Could you check a few things on this model? Use its own coordinates, in mm. Face numbers are marked on the shaded views. Round coordinates to 2 decimals unless told otherwise and drop trailing zeros. Loops run counter-clockwise (first coordinate to the right, second up) from the corner with the lowest first, then second, coordinate; pieces in that order, holes last. Notation, with made-up numbers: (-4, 27) -> (36, 27) arc R32 cw to (36, 66) -> close; hole circle Ø7 at (35.25, 0.25). An arc over 180 degrees is marked (long way). One line per item, written item: value.
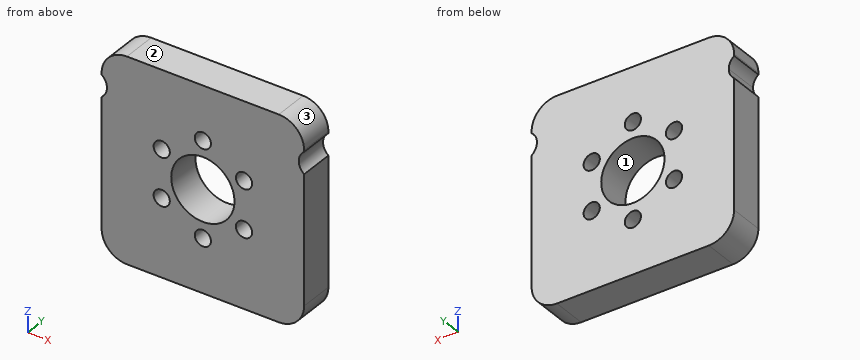
```python
from build123d import *

# Parameters (mm, degrees)
SKETCH1_R           = 6.25
BOSS_EXTRUDE1_DEPTH = 6.825
SKETCH6_R           = 1.6
CUT_EXTRUDE1_DEPTH  = 30.096058582
FILLET2_R           = 5


with BuildPart() as part:
    # Sketch1 → Boss-Extrude1 (new body)
    with BuildSketch(Plane(origin=(0, 0, 0), x_dir=(1, 0, 0), z_dir=(0, 1, 0))):
        with BuildLine():
            Line((-20, -14.645854519), (-20, -20))
            Line((-20, -20), (20, -20))
            Line((20, -20), (20, -14.645854519))
            ThreePointArc((20, -14.645854519), (18.943369346, -12.5), (20, -10.354145481))
            Line((20, -10.354145481), (20, 20))
            Line((20, 20), (-20, 20))
            Line((-20, 20), (-20, -10.354145481))
            ThreePointArc((-20, -10.354145481), (-19.221849833, -11.304052681), (-18.943369346, -12.5))
            ThreePointArc((-18.943369346, -12.5), (-19.221849833, -13.695947319), (-20, -14.645854519))
        make_face()
        with Locations(Location((0, 0, 0), (0, 0, 270))):
            Circle(SKETCH1_R, mode=Mode.SUBTRACT)
    extrude(amount=BOSS_EXTRUDE1_DEPTH)

    # Sketch6 → Cut-Extrude1 (cut, through all)
    with BuildSketch(Plane(origin=(0, 6.825, 0), x_dir=(1, 0, 0), z_dir=(0, 1, 0))):
        with Locations(Location((0, -9.385, 0), (0, 0, 270))):
            Circle(SKETCH6_R)
        with Locations(Location((-8.127648415, -4.6925, 0), (0, 0, 270))):
            Circle(SKETCH6_R)
        with Locations(Location((-8.127648415, 4.6925, 0), (0, 0, 270))):
            Circle(SKETCH6_R)
        with Locations(Location((0, 9.385, 0), (0, 0, 270))):
            Circle(SKETCH6_R)
        with Locations(Location((8.127648415, 4.6925, 0), (0, 0, 270))):
            Circle(SKETCH6_R)
        with Locations(Location((8.127648415, -4.6925, 0), (0, 0, 270))):
            Circle(SKETCH6_R)
    extrude(amount=-CUT_EXTRUDE1_DEPTH, mode=Mode.SUBTRACT)

    # Fillet2
    fillet2_edges = [part.edges().sort_by_distance(p)[0] for p in [
        (-20, 3.4125, -20),
        (20, 3.4125, -20),
        (20, 3.4125, 20),
        (-20, 3.4125, 20),
    ]]
    fillet(fillet2_edges, radius=FILLET2_R)


solid = part.part
```
Item 1: If we section it at C-C on x = 0: List the corners of the cut face in (y, z) for me (3 decimals).
Output:
outline: (0, -20) -> (6.825, -20) -> (6.825, -10.985) -> (0, -10.985) -> close; (0, -7.785) -> (6.825, -7.785) -> (6.825, -6.25) -> (0, -6.25) -> close; (0, 6.25) -> (6.825, 6.25) -> (6.825, 7.785) -> (0, 7.785) -> close; (0, 10.985) -> (6.825, 10.985) -> (6.825, 20) -> (0, 20) -> close
Item 2: If we section it at B-B on x = -5: List the corners of the cut face in (y, z) for me (3 decimals), plus the area to 3 significant figures.
Output:
outline: (0, -20) -> (6.825, -20) -> (6.825, -3.75) -> (0, -3.75) -> close; (0, 3.75) -> (6.825, 3.75) -> (6.825, 20) -> (0, 20) -> close
area: 222 mm²
Item 3: If we section it at A-A on z = 0: List the corners of the cut face in (x, y) for me (3 decimals), plus the area to 3 significant figures.
Output:
outline: (-20, 0) -> (-6.25, 0) -> (-6.25, 6.825) -> (-20, 6.825) -> close; (6.25, 0) -> (20, 0) -> (20, 6.825) -> (6.25, 6.825) -> close
area: 188 mm²
Item 4: If we mould it in two halves opening along X, with no side actions, what happens to the marked faces 1, 2 and 3? For each: released by +X, released by -X, zero draft, split by the parting line, or undercut.
Output:
face 1: undercut
face 2: zero draft
face 3: released by +X
Item 5: If we section it at D-D on y = 1.25: Count the separate pieces of the cut face and the enclosed holes in it, plus the area to 3 significant figures.
Output:
separate pieces: 1
enclosed holes: 7
area: 1,400 mm²
Item 6: I need wall thicknesses on line 1 (Z direction, x = 8, y = 3); line 2 (Z direction, x = 4, y = 5.5); line 3 (Z direction, x = 5.5, y = 2.5). Which ranges of each line are inside material? Lowest first, please. Write a range as from..to.
Output:
line 1: z = -20..-6.29, -3.1..3.1, 6.29..20
line 2: z = -20..-4.8, 4.8..20
line 3: z = -20..-2.97, 2.97..20
